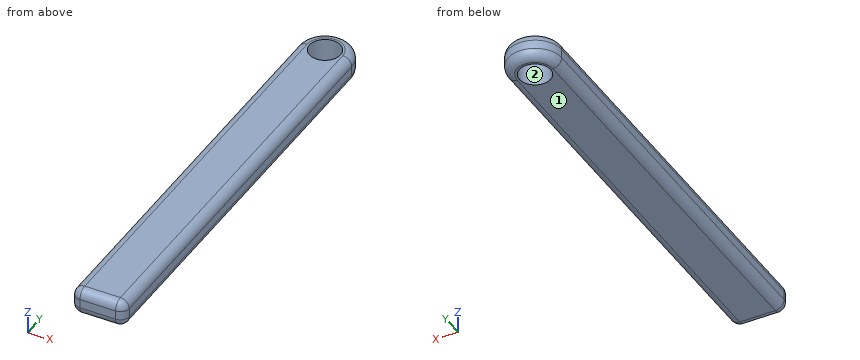
Autodesk Inventor part; units mm, degrees
ref_plane "РабПлоскость1" through (0, 0, 3) normal (0, 0, 1) x (1, 0, 0)
ref_plane "РабПлоскость2" through (0, 0, 3) normal (0, 0, 1) x (1, 0, 0)
ref_plane "YZ Plane" through (0, 0, 0) normal (1, 0, 0) x (0, 1, 0)
sketch "Эскиз1" plane through (0, 0, 0) normal (0, 0, 1) x (1, 0, 0)
  line L0 (0, 0) -> (-6, 0)
  line L1 (-6, 0) -> (-6, 47)
  line L2 (-6, 47) -> (0, 47)
  line L3 (0, 47) -> (0, 0)
  dimension "d0" = 6
  dimension "d1" = 47
extrude "Выдавливание1" add sketch "Эскиз1" along normal blind 3
fillet "Сопряжение1" radius 1 2 edges at (0, 0, 1.5) (-6, 0, 1.5)
ref_plane "РабПлоскость1" through (0, 0, 3) normal (0, 0, 1) x (1, 0, 0)
sketch "Эскиз3" plane through (0, 0, 3) normal (0, 0, 1) x (1, 0, 0)
  line L0 (0, 47) -> (-6, 47)
  circle A0 centre (-3, 47) radius 3
  point P0 (0, 0)
  dimension "d6" = 6
extrude "Выдавливание2" add sketch "Эскиз3" against normal blind 3
ref_plane "РабПлоскость2" through (0, 0, 3) normal (0, 0, 1) x (1, 0, 0)
sketch "Эскиз4" plane through (0, 0, 3) normal (0, 0, 1) x (1, 0, 0)
  circle A0 centre (-3, 47) radius 1.75
  point P0 (0, 0)
  dimension "d10" = 3.5
extrude "Выдавливание3" cut sketch "Эскиз4" against normal through all
fillet "Сопряжение2" radius 1 12 edges at (-0.2929, 0.2929, 3) (0, 24, 3) (-3, 50, 3) (-6, 24, 3) (-5.7071, 0.2929, 3) (-3, 0, 3) (-5.7071, 0.2929, 0) (-6, 24, 0) (-3, 50, 0) (0, 24, 0) (-0.2929, 0.2929, 0) (-3, 0, 0)
properties part number "ручка"
Can you work these out from the model? Positions are in its coordinate system, mm. Face numbers are marked on the shaded views. Round coordinates to 2 decimals unless told otherwise and drop trailing zeros. Loops run counter-clockwise (first coordinate to the right, second up) from the corner with the lowest first, then second, coordinate; pieces in that order, holes last. Notation, with made-up numbers: (34, -20) -> (56, -20) arc R20 ccw to (56, -1) -> close; hole circle Ø6 at (46, -17). An arc over 180 degrees is marked (long way). Answer in a Markdown table with one row per item.
Item 1: Suppose I cut it at B-B, the plane y = 7. List the corners of the cut face in (x, z) for me, plus the area to 3 significant figures.
Answer block:
| item | result |
|---|---|
| outline | (-6, 1) arc R1 ccw to (-5, 0) -> (-1, 0) arc R1 ccw to (0, 1) -> (0, 2) arc R1 ccw to (-1, 3) -> (-5, 3) arc R1 ccw to (-6, 2) -> close |
| area | 17.1 mm² |
Item 2: Will this pin go through, and if not, where does the flat tip stop? P1, Ø1.5, axis at x = -4, z = 0.5, coming from the +Y side.
Answer block:
| item | result |
|---|---|
| P1 | y = 49.97 |
Item 3: We'd pull the mould along X, two halves only. Please class the marked faces 1 and 2: released by +X, released by -X, zero draft, split by the parting line, or undercut.
Answer block:
| item | result |
|---|---|
| face 1 | zero draft |
| face 2 | undercut |
Item 4: If I drill on probe 1 along Y at (x, z) = (-3, 1.95); probe 2 along Y at (x, z) = (-1.5, 2.7); probe 3 along X at (y, z) = (17, 2.25), over which ranges is the centre line in solid material (lowest first)?
Answer block:
| item | result |
|---|---|
| probe 1 | 0 to 45.25, 48.75 to 50 |
| probe 2 | 0.29 to 46.1, 47.9 to 49.26 |
| probe 3 | -5.97 to -0.03 |
Item 5: Suppose I cut it at A-A, the plane x = -3. List the corners of the cut face in (y, z) for me.
Answer block:
| item | result |
|---|---|
| outline | (0, 1) arc R1 ccw to (1, 0) -> (45.25, 0) -> (45.25, 3) -> (1, 3) arc R1 ccw to (0, 2) -> close; (48.75, 0) -> (49, 0) arc R1 ccw to (50, 1) -> (50, 2) arc R1 ccw to (49, 3) -> (48.75, 3) -> close |
